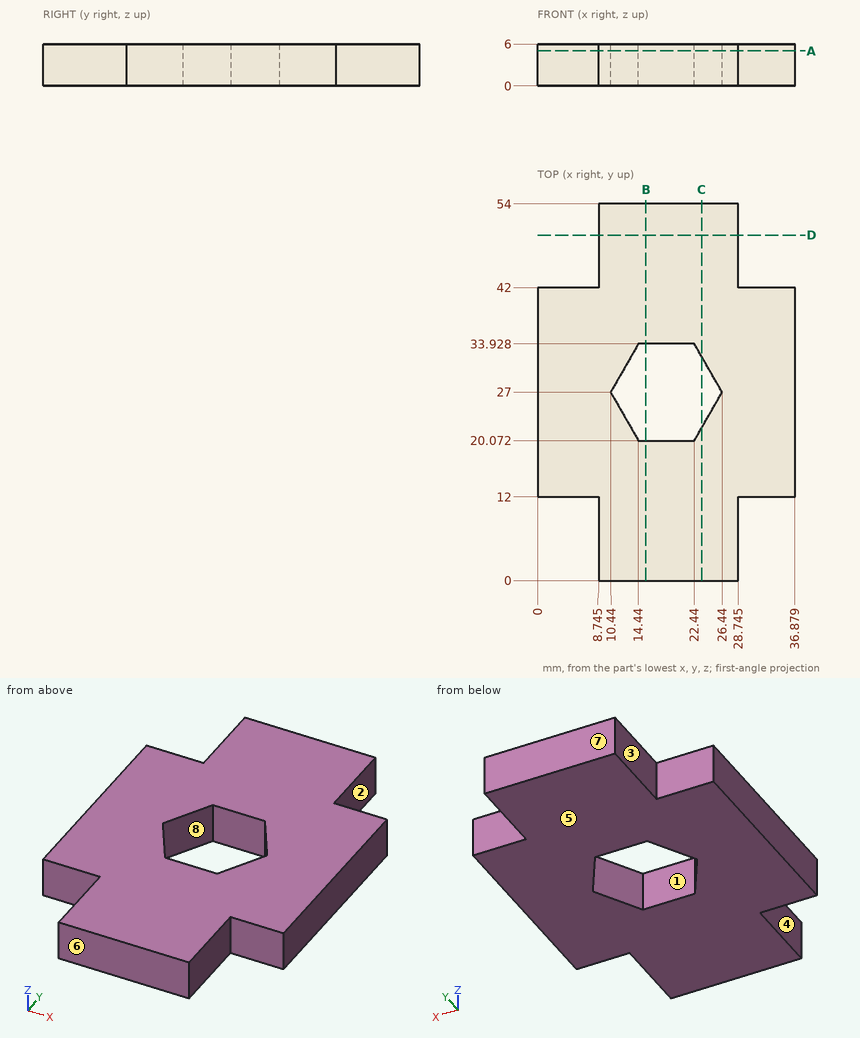
Geometry: see drawing. Coordinates: mm, zero at the bounding-box minimum. A direction names the side the tool comes from. Round coordinates to 2 decimals unless told otherwise and drop trailing zeros. Loops run counter-clockwise (first coordinate to the right, second up) from the corner with the lowest first, then second, coordinate; pieces in that order, holes last. Notation, with made-up numbers: M 8.25,83.5 L 49.25,83.5 A23 cw 49.25,95.5 Z; hole C 29,33 d1. An arc over 180 degrees is marked long. Use a Markdown table: item, result. Add a question column.
1. Section query A-A on z = 5. Return the cut outline in (x, y) (1 decimal), then the cut area to 3 significant figures.
2. Section query C-C on x = 23.5. Return the cut outline in (y, z).
3. Line query: line 1 (Y direction, x = 17, z = 4.25); line 2 (Y direction, x = 13.5, z = 4.6); line 3 (X direction, y = 5, z = 0.6) (1 decimal). Output: solid intervals per line, ascending.
4. Section query B-B on x = 15.5. Return the cut outline in (y, z), then the cut area to 3 significant figures.
5. Mould query, pull axis Y, two halves, no side actions, for the marked faces 5, 6, 7 and 8. Classes: pulls with the +Y half, pulls with the -Y half, needs draft (parallel to the pull), parting line crosses it, or undercut.
6. Contact query for flat-ended pins moving along their axis: P1, Ø1.8, axis at x = 3.5, z = 2, coming from the +Y side; P2, Ø1.8, axis at y = 46.5, z = 1.5, coming from the +X side (3 decimals); P3, Ø3, axis at x = 3.5, z = 2.5, coming from the -Y side. Output: stop coordinate, or through.
7. Reachability of the marked faces 1, 2, 3 and 4 from +Z, -Z, +X, -X, +Y, -Y: full face, straight path, thin tool, end or side. Return the list, or none.
8. Section query D-D on y = 49.5. Return the cut outline in (x, z) (1 decimal), then the cut area to 3 significant figures.
Reported:
| question | item | result |
|---|---|---|
| 1 | outline | M 0,12 L 8.7,12 L 8.7,0 L 28.7,0 L 28.7,12 L 36.9,12 L 36.9,42 L 28.7,42 L 28.7,54 L 8.7,54 L 8.7,42 L 0,42 Z; hole M 10.4,27 L 14.4,20.1 L 22.4,20.1 L 26.4,27 L 22.4,33.9 L 14.4,33.9 Z |
| 1 | area | 1,420 mm² |
| 2 | outline | M 0,0 L 21.91,0 L 21.91,6 L 0,6 Z; M 32.09,0 L 54,0 L 54,6 L 32.09,6 Z |
| 3 | line 1 | y = 0 to 20.07, 33.93 to 54 |
| 3 | line 2 | y = 0 to 21.7, 32.3 to 54 |
| 3 | line 3 | x = 8.7 to 28.7 |
| 4 | outline | M 0,0 L 20.07,0 L 20.07,6 L 0,6 Z; M 33.93,0 L 54,0 L 54,6 L 33.93,6 Z |
| 4 | area | 241 mm² |
| 5 | face 5 | needs draft |
| 5 | face 6 | pulls with the -Y half |
| 5 | face 7 | pulls with the +Y half |
| 5 | face 8 | undercut |
| 6 | P1 | stops at y = 42 |
| 6 | P2 | stops at x = 28.745 |
| 6 | P3 | stops at y = 12 |
| 7 | face 1 | +Z, -Z |
| 7 | face 2 | +Z, -Z, +X, +Y |
| 7 | face 3 | +Z, -Z, -X, +Y |
| 7 | face 4 | +Z, -Z, -X, -Y |
| 8 | outline | M 8.7,0 L 28.7,0 L 28.7,6 L 8.7,6 Z |
| 8 | area | 120 mm² |
